Build history of the part. All positions in model axes, mm. Face numbers are marked on the shaded views. Give positions to 0.01 mm unless a question says otherwise; leave off trailing zeros. Order: outer loops, then holes, each group sorted by start corner. A loop starts at its lowest first (then second) coordinate and runs counter-clockwise, first axis right, second up. Notation, with made-up numbers: M 79,5 L 86,5 A15 cw 86,19 Z; hole C 12,38.25 d9. An arc over 180 degrees is marked long. One line per item, written item: value.
from build123d import *

# Parameters (mm, degrees)
BOSS_EXTRU_1_DEPTH                             = 15
FRAISAGE_POUR_VIS_T_TE_FRAIS_E_M51_D           = 5.5
FRAISAGE_POUR_VIS_T_TE_FRAIS_E_M51_CSINK_D     = 10.4
FRAISAGE_POUR_VIS_T_TE_FRAIS_E_M51_CSINK_ANGLE = 90
CONG_2_R                                       = 5


with BuildPart() as part:
    # Esquisse1 → Boss.-Extru.1 (new body)
    with BuildSketch(Plane(origin=(0, 0, 0), x_dir=(1, 0, 0), z_dir=(0, 1, 0))):
        Polygon((-17.5, 109.5), (-27.5, 12.5), (-27.5, -12.5), (-17.5, -109.5), (17.5, -109.5), (27.5, -12.5), (27.5, 12.5), (17.5, 109.5), align=None)
    extrude(amount=BOSS_EXTRU_1_DEPTH)

    # Fraisage pour vis à tête fraisée M51 (through all)
    with Locations(Plane(origin=(0, 15, 0), x_dir=(1, 0, 0), z_dir=(0, 1, 0))):
        with Locations((-7.5, 30), (7.5, 30), (7.5, 15), (-7.5, 15), (-7.5, 0), (7.5, 0), (7.5, -15), (-7.5, -15), (-7.5, -30), (7.5, -30), (0, -94.5), (0, 94.5)):
            CounterSinkHole(FRAISAGE_POUR_VIS_T_TE_FRAIS_E_M51_D / 2, FRAISAGE_POUR_VIS_T_TE_FRAIS_E_M51_CSINK_D / 2, counter_sink_angle=FRAISAGE_POUR_VIS_T_TE_FRAIS_E_M51_CSINK_ANGLE)

    # Congé2
    cong_2_edges = [part.edges().sort_by_distance(p)[0] for p in [
        (27.5, 7.5, -12.5),
        (27.5, 7.5, 12.5),
        (17.5, 7.5, 109.5),
        (-17.5, 7.5, 109.5),
        (-27.5, 7.5, 12.5),
        (-27.5, 7.5, -12.5),
        (-17.5, 7.5, -109.5),
        (17.5, 7.5, -109.5),
    ]]
    fillet(cong_2_edges, radius=CONG_2_R)


solid = part.part
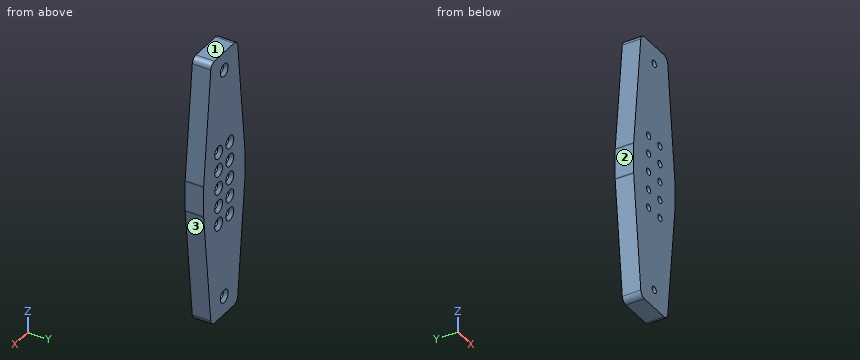
1) Pin check, flat tips, straight feed: pin 1 (2 mm diameter, centred on y = 9.5, z = 23.5, fed in from -X); pin 2 (7 mm diameter, centred on x = 0, z = -94.5, fed in from +Y); pin 3 (3.5 mm diameter, centred on x = 7.5, z = -15, fed in from +Y); pin 4 (1.5 mm diameter, centred on y = 11.5, z = -62, fed in from -X). Stop position of each tip, or through.
Check values:
pin 1: x = -26.47
pin 2: y = 13.3
pin 3: through
pin 4: x = -22.47
2) Mould opens along X. For the marked faces 1, 2 and 3 say: released by +X, released by -X, zero draft, split by the parting line, or undercut.
Check values:
face 1: zero draft
face 2: released by -X
face 3: released by +X
3) Saw through at C-C, the plane z = 15. Write the cut outline in (x, y), then the cut area to 3 significant figures.
Check values:
outline: M -27.24,0 L -10.25,0 L -10.25,12.55 L -12.7,15 L -27.24,15 Z; M -4.75,0 L 4.75,0 L 4.75,12.55 L 2.3,15 L -2.3,15 L -4.75,12.55 Z; M 10.25,0 L 27.24,0 L 27.24,15 L 12.7,15 L 10.25,12.55 Z
area: 640 mm^2
4) Saw through at D-D, the plane x = -20. Write the cut outline in (y, z).
Check values:
outline: M 0,-85.25 L 15,-85.25 L 15,85.25 L 0,85.25 Z
5) Saw through at A-A, the plane x = 7.5. Give the number of separate pieces and of enclosed holes in the cut face, then the cut area to 3 significant figures.
Check values:
separate pieces: 6
enclosed holes: 0
area: 2,840 mm^2
6) Drill centre lines: probe 1 along X at (y, z) = (10, 15); probe 2 along X at (y, z) = (3.75, -30); probe 3 along Z at (x, y) = (5, 5.75). Where is each one in solid material? Low to high. Write a range as from..to.
Check values:
probe 1: -27.24..-10.25, -4.75..4.75, 10.25..27.24
probe 2: -25.7..-10.25, -4.75..4.75, 10.25..25.7
probe 3: -109.5..-31.15, -28.85..-16.15, -13.85..-1.15, 1.15..13.85, 16.15..28.85, 31.15..109.5
